```python
from build123d import *

# Parameters (mm, degrees)
ESQUISSE2_OUTSIDE_W     = 14.638
ESQUISSE2_OUTSIDE_H     = 14.638
ENL_V_MAT_EXTRU_1_DEPTH = 10
CHANFREIN1_SIZE         = 0.5


with BuildPart() as part:
    # Esquisse1 → Révolution1 (revolve)
    with BuildSketch(Plane.XY, mode=Mode.PRIVATE) as r_volution1_sk:
        Polygon((1.25, 0.2), (2, 0.95), (13, 0.95), (13, 3), (9, 3), (9, 2.5), (8, 2.5), (8, 4.5), (4, 4.5), (0, 0.5), (0, 0.2), align=None)
    revolve(r_volution1_sk.sketch.rotate(Axis((0, 0, 0), (1, 0, 0)), 90), axis=Axis((0, 0, 0), (1, 0, 0)))

    # Esquisse2 outside → Enlèv. mat.-Extru.1 (cut)
    with BuildSketch(Plane(origin=(8, 0, 0), x_dir=(0, 0, -1), z_dir=(1, 0, 0))):
        Rectangle(ESQUISSE2_OUTSIDE_W, ESQUISSE2_OUTSIDE_H)
        Polygon((-3.5, -2.020725942), (0, -4.041451884), (3.5, -2.020725942), (3.5, 2.020725942), (0, 4.041451884), (-3.5, 2.020725942), align=None, mode=Mode.SUBTRACT)
    extrude(amount=-ENL_V_MAT_EXTRU_1_DEPTH, mode=Mode.SUBTRACT)

    # Chanfrein1
    chanfrein1_edges = [part.edges().sort_by_distance(p)[0] for p in [
        (9, 0, -3),
        (13, 0, -3),
    ]]
    chamfer(chanfrein1_edges, length=CHANFREIN1_SIZE - 0.0001)  # a hair under: the kernel refuses the full size


solid = part.part
```
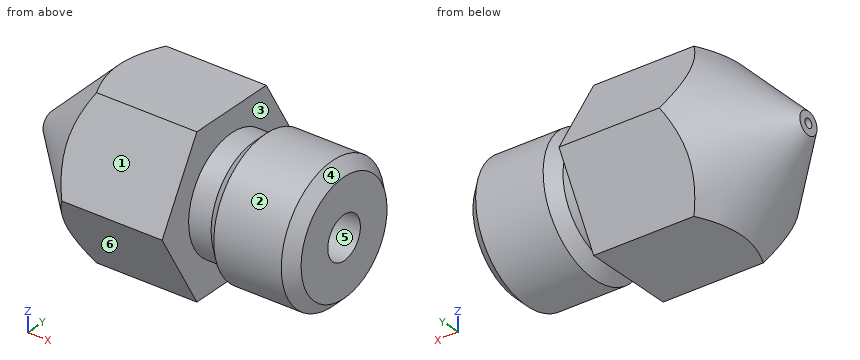
Design review of the part built by this model. Coordinates are the model's own, in mm. Face numbers are marked on the shaded views. A direction names the side the tool comes from. Coordinates: 2 decimals unless noted, no trailing zeros. Order: outer loops, then holes, each group sorted by start corner. A loop starts at its lowest first (then second) coordinate and runs counter-clockwise, first axis right, second up. Notation, with made-up numbers: (86.25, 19.25) - (110.25, 19.25) arc R33 cw to (110.25, 57.25) - close; hole circle Ø5 at (-36, 35). An arc over 180 degrees is marked (long way). Answer in a Markdown table with one row per item.
(1) Consider section B-B on x = 4.5. State the section outline as (y, z) points.
Checked values:
| item | result |
|---|---|
| outline | (-4.04, 0) - (-2.02, -3.5) - (2.02, -3.5) - (4.04, 0) - (2.02, 3.5) - (-2.02, 3.5) - close; hole circle Ø1.9 at (0, 0) |
(2) Wall thickness on line 1 along Y through (x, z) = (11.25, 0); line 2 along X through (y, z) = (-0.75, -2.75); line 3 along Y through (x, z) = (4, 0.25): over which ranges is each line inside the solid? List them lowest first. Write a range as from..to.
Checked values:
| item | result |
|---|---|
| line 1 | -3..-0.95, 0.95..3 |
| line 2 | 2.35..8, 9.35..12.65 |
| line 3 | -3.9..-0.92, 0.92..3.9 |
(3) Consider section C-C on x = 12.25. State the section outline as (y, z) points, plus the area to 3 significant figures.
Checked values:
| item | result |
|---|---|
| outline | circle Ø6 at (0, 0); hole circle Ø1.9 at (0, 0) |
| area | 25.4 mm^2 |
(4) The part is to be moulded in two halves that separate along Z. For the marked faces 4, 5 and 6, say which applies: released by +Z, released by -Z, zero draft, split by the parting line, or undercut.
Checked values:
| item | result |
|---|---|
| face 4 | split by the parting line |
| face 5 | undercut |
| face 6 | released by -Z |
(5) For the marked faces 1, 2 and 3, list the 3-axis set-ups (+Z, -Z, +X, -X, +Y, -Y) from which the entire face can be reached by the end or side of a thin tool; tool diameter is ignored.
Checked values:
| item | result |
|---|---|
| face 1 | +Z, +X, -X, -Y |
| face 2 | +X |
| face 3 | none |
(6) Clearance check with flat-ended pins moving along their axes: pin 1 (2 mm diameter, centred on x = 9.5, y = -2.5, fed in from +Z); pin 2 (3 mm diameter, centred on y = 1.5, z = -1.5, fed in from -X); pin 3 (4 mm diameter, centred on x = 10, y = -3, fed in from -Z). State where each tip first meets the part, or that it passes through.
Checked values:
| item | result |
|---|---|
| pin 1 | z = 2.6 |
| pin 2 | x = 0.12 |
| pin 3 | z = -2.83 |
